Could you check a few things on this model? Use its own coordinates, in mm. Face numbers are marked on the shaded views. A direction names the side the tool comes from. Give positions to 0.01 mm unless a question says otherwise; leave off trailing zeros. Write each loop counter-clockwise with the first axis right and the second up, starting at its lowest first coordinate (ties: lowest second). Pieces come first, ordered by that corner, then holes. Notation, with made-up numbers: M -14.75,40.25 L 35.25,40.25 A19 cw 35.25,59.25 Z; hole C 53.5,-24.5 d2. An arc over 180 degrees is marked long. Use one line per item in the form item = value.
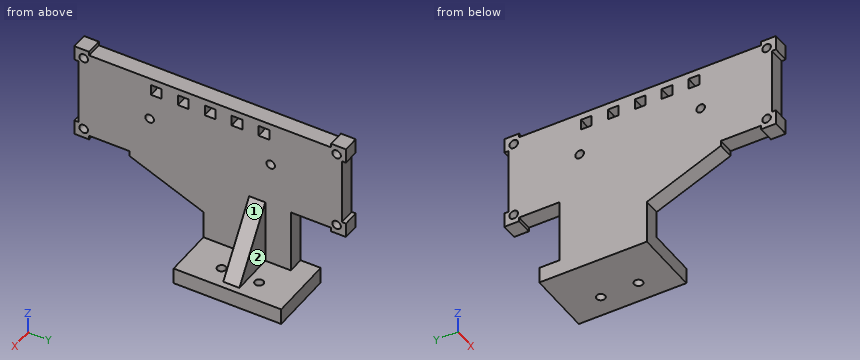
from build123d import *

# Parameters (mm, degrees)
EXTRUDE_1_DEPTH     = 6
SKETCH_2_R          = 1.6
CUT_EXTRUDE_1_DEPTH = 6
SKETCH_3_W          = 26
SKETCH_3_H          = 60
CUT_EXTRUDE_2_DEPTH = 6
SKETCH_4_W          = 4
SKETCH_4_H          = 4
CUT_EXTRUDE_3_DEPTH = 6
SKETCH_5_W          = 24.42858663
SKETCH_5_H          = 75.5
EXTRUDE_2_DEPTH     = 6
SKETCH_6_W          = 6
SKETCH_6_H          = 60
EXTRUDE_3_DEPTH     = 54.343929089
SKETCH_7_R          = 1.6
CUT_EXTRUDE_4_DEPTH = 6
SKETCH_8_R          = 1.6
CUT_EXTRUDE_5_DEPTH = 6
EXTRUDE_5_DEPTH     = 6
SKETCH_15_W         = 30
SKETCH_15_H         = 60
CUT_EXTRUDE_6_DEPTH = 20
SKETCH_16_W         = 30
SKETCH_16_H         = 30
CUT_EXTRUDE_7_DEPTH = 20
CUT_EXTRUDE_8_DEPTH = 10


with BuildPart() as part:
    # Sketch 1 → Extrude 1 (new body)
    with BuildSketch(Plane(origin=(193.15, 0, 0), x_dir=(0, 0, -1), z_dir=(1, 0, 0))):
        Polygon((-82, -62.5), (-82, -68), (-87.5, -68), (-87.5, -66.5), (-112.5, -66.5), (-112.5, -68), (-118, -68), (-118, -62.5), (-116.5, -62.5), (-116.5, 27.5), (-118, 27.5), (-118, 33), (-112.5, 33), (-112.5, 31.5), (-87.5, 31.5), (-87.5, 33), (-82, 33), (-82, 27.5), (-83.5, 27.5), (-83.5, -62.5), align=None)
    extrude(amount=EXTRUDE_1_DEPTH)

    # Sketch 2 → Cut-Extrude 1 (cut)
    with BuildSketch(Plane(origin=(193.15, 0, 0), x_dir=(0, 0, -1), z_dir=(1, 0, 0))):
        with Locations((-85.5, -64.5)):
            Circle(SKETCH_2_R)
        with Locations((-114.5, -64.5)):
            Circle(SKETCH_2_R)
        with Locations((-85.5, 29.5)):
            Circle(SKETCH_2_R)
        with Locations((-114.5, 29.5)):
            Circle(SKETCH_2_R)
    extrude(amount=CUT_EXTRUDE_1_DEPTH, mode=Mode.SUBTRACT)

    # Sketch 3 → Cut-Extrude 2 (cut)
    with BuildSketch(Plane(origin=(193.15, 0, 0), x_dir=(0, 0, -1), z_dir=(1, 0, 0))):
        with Locations((-94, -17.5)):
            Rectangle(SKETCH_3_W, SKETCH_3_H)
    extrude(amount=CUT_EXTRUDE_2_DEPTH, mode=Mode.SUBTRACT)

    # Sketch 4 → Cut-Extrude 3 (cut)
    with BuildSketch(Plane(origin=(193.15, 0, 0), x_dir=(0, 0, -1), z_dir=(1, 0, 0))):
        with Locations((-112, -37.5)):
            Rectangle(SKETCH_4_W, SKETCH_4_H)
        with Locations((-112, -27.5)):
            Rectangle(SKETCH_4_W, SKETCH_4_H)
        with Locations((-112, -17.5)):
            Rectangle(SKETCH_4_W, SKETCH_4_H)
        with Locations((-112, -7.5)):
            Rectangle(SKETCH_4_W, SKETCH_4_H)
        with Locations((-112, 2.5)):
            Rectangle(SKETCH_4_W, SKETCH_4_H)
    extrude(amount=CUT_EXTRUDE_3_DEPTH, mode=Mode.SUBTRACT)



with BuildPart() as body_2:
    # Sketch 5 → Extrude 2 (new body)
    with BuildSketch(Plane.XY.offset(53.656070911)):
        with Locations((205.364293315, -9.75)):
            Rectangle(SKETCH_5_W, SKETCH_5_H)
    extrude(amount=EXTRUDE_2_DEPTH)


with BuildPart() as part_1:
    add(part.part)

    add(body_2.part)  # Extrude 3 merges body 2
    # Sketch 6 → Extrude 3 (add)
    with BuildSketch(Plane.XY.offset(53.656070911)):
        with Locations((196.15, -17.5)):
            Rectangle(SKETCH_6_W, SKETCH_6_H)
    extrude(amount=EXTRUDE_3_DEPTH)

    # Sketch 7 → Cut-Extrude 4 (cut)
    with BuildSketch(Plane.XY.offset(59.656070911)):
        with Locations((209.57858663, -7)):
            Circle(SKETCH_7_R)
        with Locations((209.57858663, 7)):
            Circle(SKETCH_7_R)
    extrude(amount=-CUT_EXTRUDE_4_DEPTH, mode=Mode.SUBTRACT)

    # Sketch 8 → Cut-Extrude 5 (cut)
    with BuildSketch(Plane(origin=(199.15, 0, 0), x_dir=(0, 0, -1), z_dir=(1, 0, 0))):
        with Locations((-100, -40)):
            Circle(SKETCH_8_R)
        with Locations((-100, 5)):
            Circle(SKETCH_8_R)
    extrude(amount=-CUT_EXTRUDE_5_DEPTH, mode=Mode.SUBTRACT)

    # Sketch 10 → Extrude 5 (add)
    with BuildSketch(Plane(origin=(0, -3, 0), x_dir=(1, 0, 0), z_dir=(0, 1, 0))):
        Polygon((199.15, -59.656070911), (215.15, -59.656070911), (199.15, -83.656070911), align=None)
    extrude(amount=EXTRUDE_5_DEPTH)

    # Sketch 15 → Cut-Extrude 6 (cut)
    with BuildSketch(Plane.XY.offset(50)):
        with Locations((205, -50)):
            Rectangle(SKETCH_15_W, SKETCH_15_H)
    extrude(amount=CUT_EXTRUDE_6_DEPTH, mode=Mode.SUBTRACT)

    # Sketch 16 → Cut-Extrude 7 (cut)
    with BuildSketch(Plane.XY.offset(50)):
        with Locations((205, 35)):
            Rectangle(SKETCH_16_W, SKETCH_16_H)
    extrude(amount=CUT_EXTRUDE_7_DEPTH, mode=Mode.SUBTRACT)

    # Sketch 17 → Cut-Extrude 8 (cut)
    with BuildSketch(Plane(origin=(190, 0, 0), x_dir=(0, 0, -1), z_dir=(1, 0, 0))):
        Polygon((-70, -47.5), (-81.5, -47.5), (-70, -20), align=None)
    extrude(amount=CUT_EXTRUDE_8_DEPTH, mode=Mode.SUBTRACT)


solid = part_1.part
1) I want a section at D-D, the plane x = 209.75. Please give me the cut outline in (y, z).
Checked values:
outline = M -20,53.66 L -8.59,53.66 L -8.59,59.66 L -20,59.66 Z; M -5.41,53.66 L 5.41,53.66 L 5.41,59.66 L 3,59.66 L 3,67.76 L -3,67.76 L -3,59.66 L -5.41,59.66 Z; M 8.59,53.66 L 20,53.66 L 20,59.66 L 8.59,59.66 Z
2) If I drill on L1, parallel to Y at x = 197.9, z = 100; L2, parallel to Y at x = 197.4, z = 85.5; L3, parallel to Z at x = 195.5, y = 17, over which ranges is the centre line in solid material (lowest first)?
Checked values:
L1 = -66.5 to -41.6, -38.4 to 3.4, 6.6 to 31.5
L2 = -68 to -66.1, -62.9 to 27.9, 31.1 to 33
L3 = 53.66 to 59.66, 83.5 to 116.5
3) I want a section at B-B, the plane z = 85.5. Please give me the cut outline in (x, y).
Checked values:
outline = M 193.15,-68 L 199.15,-68 L 199.15,-66.1 L 193.15,-66.1 Z; M 193.15,-62.9 L 199.15,-62.9 L 199.15,27.9 L 193.15,27.9 Z; M 193.15,31.1 L 199.15,31.1 L 199.15,33 L 193.15,33 Z
4) I want a section at A-A, the plane y = 1.5. Please give me the cut outline in (x, z), plus the area to 3 significant figures.
Checked values:
outline = M 193.15,53.66 L 217.58,53.66 L 217.58,59.66 L 215.15,59.66 L 199.15,83.66 L 199.15,110 L 193.15,110 Z; M 193.15,114 L 199.15,114 L 199.15,116.5 L 193.15,116.5 Z
area = 656 mm2
5) I want a section at C-C, the plane y = 29.5. Please give me the cut outline in (x, z).
Checked values:
outline = M 193.15,82 L 199.15,82 L 199.15,83.9 L 193.15,83.9 Z; M 193.15,87.1 L 199.15,87.1 L 199.15,112.9 L 193.15,112.9 Z; M 193.15,116.1 L 199.15,116.1 L 199.15,118 L 193.15,118 Z
6) For the marked faces 1 and 2, which set-ups out of +Z, -Z, +X, -X, +Y, -Y let a thin tool reach every point of the face, with its end or its side?
Checked values:
face_1 = +Z, +X, +Y, -Y
face_2 = +Z, +X, +Y
7) For pin 1 Ø10 at (x, y) = (195.5, -9.5) entering from +Z; pin 2 Ø3 at (x, z) = (201.5, 62.5) entering from -Y; pin 3 Ø0.8 at (x, y) = (195, -67.5) entering from -Z, each with a flat end and sliding along its axis, tell me the tip position at first contact or that it passes through.
Checked values:
pin_1 = 116.5
pin_2 = -3
pin_3 = 82
